```python
from build123d import *


with BuildPart() as part:
    # Esboço1 → Revolução1 (revolve)
    with BuildSketch(Plane.XY, mode=Mode.PRIVATE) as revolu_o1_sk:
        Polygon((5, 0), (5, -30), (27.5, -30), (27.5, -14), (25.5, -12), (25.5, -8), (27.5, -6), (27.5, 0), align=None)
    revolve(revolu_o1_sk.sketch.rotate(Axis((0, 0, 0), (0, -1, 0)), 180), axis=Axis((0, 0, 0), (0, -1, 0)))  # turned: the seam where the file's is


solid = part.part
```
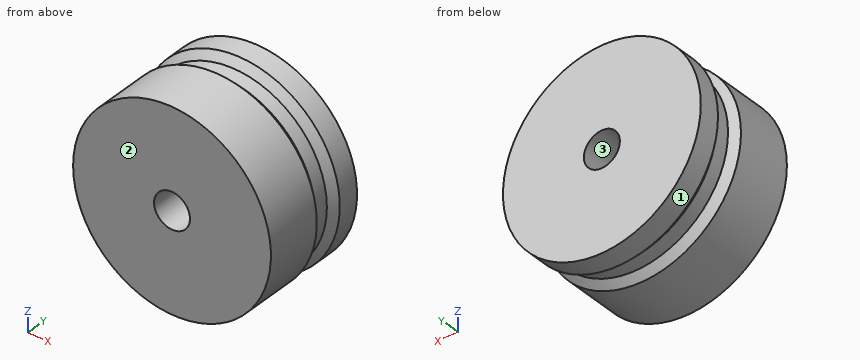
Work out the finished part from the listing and answer in its coordinate system (mm). Face numbers are marked on the shaded views. Coordinates: 2 decimals unless noted, no trailing zeros. Loops run counter-clockwise (first coordinate to the right, second up) from the corner with the lowest first, then second, coordinate; pieces in that order, holes last.
1) Section C-C (y = -24.25) is taken. Give the vertices of the cut face in (x, z).
Results:
outline: circle Ø55 at (0, 0); hole circle Ø10 at (0, 0)
2) Consider probe 1 along Z at (x, y) = (0, -22); probe 2 along Y at (x, z) = (13.5, -22.5); probe 3 along X at (y, z) = (-1.5, 1.5). Determine where each line is inside the solid, lowest interval first.
Results:
probe 1: z = -27.5 to -5, 5 to 27.5
probe 2: y = -30 to -12.74, -7.26 to 0
probe 3: x = -27.46 to -4.77, 4.77 to 27.46
3) Section A-A (z = 0) is taken. Give the vertices of the cut face in (x, y).
Results:
outline: (-27.5, -30) - (-5, -30) - (-5, 0) - (-27.5, 0) - (-27.5, -6) - (-25.5, -8) - (-25.5, -12) - (-27.5, -14) - close; (5, -30) - (27.5, -30) - (27.5, -14) - (25.5, -12) - (25.5, -8) - (27.5, -6) - (27.5, 0) - (5, 0) - close
4) Flat-ended cylindrical pins translate along their axes: pin 1 (5 mm diameter, centred on y = -24, z = 6, fed in from +X); pin 2 (1 mm diameter, centred on x = -21, y = -17, fed in from -Z); pin 3 (12 mm diameter, centred on y = -15, z = -16.5, fed in from -X). Find the tip coordinate at first contact, or state that the pin passes through.
Results:
pin 1: stops at x = 27.28
pin 2: stops at z = -18.33
pin 3: stops at x = -25.42
5) Section B-B (x = 0) is taken. Give the vertices of the cut face in (y, z).
Results:
outline: (-30, -27.5) - (-14, -27.5) - (-12, -25.5) - (-8, -25.5) - (-6, -27.5) - (0, -27.5) - (0, -5) - (-30, -5) - close; (-30, 5) - (0, 5) - (0, 27.5) - (-6, 27.5) - (-8, 25.5) - (-12, 25.5) - (-14, 27.5) - (-30, 27.5) - close
6) For a pull along Z with two mould halves and no side action, classify the marked faces 1, 2 and 3 as +Z half, -Z half, draft (parallel to the pull), parting line (faces both ways), or undercut.
Results:
face 1: parting line
face 2: draft
face 3: undercut
